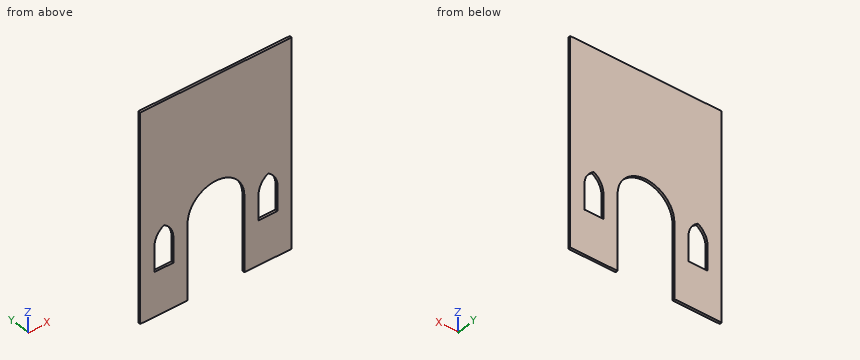
```python
from build123d import *

# Parameters (mm, degrees)
F0_W     = 1219.2
F0_H     = 1676.4
F1_DEPTH = 19.05
F3_DEPTH = 19.051
F5_DEPTH = 19.051


with BuildPart() as f1:
    # F0 (on Front) → F1 (new body)
    with BuildSketch(Plane.XZ):
        Rectangle(F0_W, F0_H)
    extrude(amount=F1_DEPTH)

    # F2 (on face) → F3 (cut, through all)
    with BuildSketch(Plane.XZ.offset(19.05)):
        with BuildLine():
            Line((-228.6, -228.6), (-228.6, -838.2))
            Line((-228.6, -838.2), (228.6, -838.2))
            Line((228.6, -838.2), (228.6, -228.6))
            ThreePointArc((228.6, -228.6), (0, 0), (-228.6, -228.6))
        make_face()
    extrude(amount=-F3_DEPTH, mode=Mode.SUBTRACT)

    # F4 (on face) → F5 (cut, through all)
    with BuildSketch(Plane.XZ.offset(19.05)):
        with BuildLine():
            Line((-495.3, -482.6), (-342.9, -482.6))
            Line((-342.9, -482.6), (-342.9, -279.4))
            ThreePointArc((-342.9, -279.4), (-363.317728, -203.2), (-419.1, -147.417728))
            ThreePointArc((-419.1, -147.417728), (-474.882272, -203.2), (-495.3, -279.4))
            Line((-495.3, -279.4), (-495.3, -482.6))
        make_face()
        with BuildLine():
            ThreePointArc((419.1, -147.417728), (363.317728, -203.2), (342.9, -279.4))
            Line((342.9, -279.4), (342.9, -482.6))
            Line((342.9, -482.6), (495.3, -482.6))
            Line((495.3, -482.6), (495.3, -279.4))
            ThreePointArc((495.3, -279.4), (474.882272, -203.2), (419.1, -147.417728))
        make_face()
    extrude(amount=-F5_DEPTH, mode=Mode.SUBTRACT)


solid = f1.part
```
Source: CAD feature listing. Evaluate the final solid. Frame: model axes, mm. Round coordinates to 2 decimals unless told otherwise and drop trailing zeros. Order: outer loops, then holes, each group sorted by start corner. A loop starts at its lowest first (then second) coordinate and runs counter-clockwise, first axis right, second up. Notation, with made-up numbers: (-16, 3.5) -> (28, 3.5) arc R25 ccw to (28, 39.5) -> close; hole circle Ø5 at (28, 18.5). An arc over 180 degrees is marked (long way). Use CSV: the item, a comma, the result in double quotes.
(1) Section A-A on z = -364. Return the cut outline in (x, y).
Report:
outline,"(-609.6, -19.05) -> (-495.3, -19.05) -> (-495.3, 0) -> (-609.6, 0) -> close; (-342.9, -19.05) -> (-228.6, -19.05) -> (-228.6, 0) -> (-342.9, 0) -> close; (228.6, -19.05) -> (342.9, -19.05) -> (342.9, 0) -> (228.6, 0) -> close; (495.3, -19.05) -> (609.6, -19.05) -> (609.6, 0) -> (495.3, 0) -> close"
(2) Section B-B on y = -7.75. Return the cut outline in (x, z).
Report:
outline,"(-609.6, -838.2) -> (-228.6, -838.2) -> (-228.6, -228.6) arc R228.6 cw to (228.6, -228.6) -> (228.6, -838.2) -> (609.6, -838.2) -> (609.6, 838.2) -> (-609.6, 838.2) -> close; hole (-495.3, -482.6) -> (-342.9, -482.6) -> (-342.9, -279.4) arc R152.4 ccw to (-419.1, -147.42) arc R152.4 ccw to (-495.3, -279.4) -> close; hole (342.9, -482.6) -> (495.3, -482.6) -> (495.3, -279.4) arc R152.4 ccw to (419.1, -147.42) arc R152.4 ccw to (342.9, -279.4) -> close"
(3) Ray query, L1, parallel to X at y = -16, z = -388.5; L2, parallel to X at y = -12.75, z = -268.5; L3, parallel to X at y = -11.5, z = -656. Return the intervals inside material, ascending.
Report:
L1,"-609.6 to -495.3, -342.9 to -228.6, 228.6 to 342.9, 495.3 to 609.6"
L2,"-609.6 to -494.91, -343.29 to -228.6, 228.6 to 343.29, 494.91 to 609.6"
L3,"-609.6 to -228.6, 228.6 to 609.6"
(4) First-contact query: pin 1 Ø1 at (x, y) = (-179, -10) entering from -Z; pin 2 Ø10 at (x, z) = (219.5, -573) entering from +Y. Flat tips, straight axial feed; report the tip coordinate or a pass-through.
Report:
pin 1,"z = -87.05"
pin 2,"through"
(5) Section D-D on z = -192.5. Return the cut outline in (x, y), and give its area (3 significant figures).
Report:
outline,"(-609.6, -19.05) -> (-468.1, -19.05) -> (-468.1, 0) -> (-609.6, 0) -> close; (-370.1, -19.05) -> (-225.73, -19.05) -> (-225.73, 0) -> (-370.1, 0) -> close; (225.73, -19.05) -> (370.1, -19.05) -> (370.1, 0) -> (225.73, 0) -> close; (468.1, -19.05) -> (609.6, -19.05) -> (609.6, 0) -> (468.1, 0) -> close"
area,"10,900 mm^2"
(6) Section C-C on x = 360. Return the cut outline in (y, z).
Report:
outline,"(-19.05, -838.2) -> (0, -838.2) -> (0, -482.6) -> (-19.05, -482.6) -> close; (-19.05, -209.26) -> (0, -209.26) -> (0, 838.2) -> (-19.05, 838.2) -> close"
